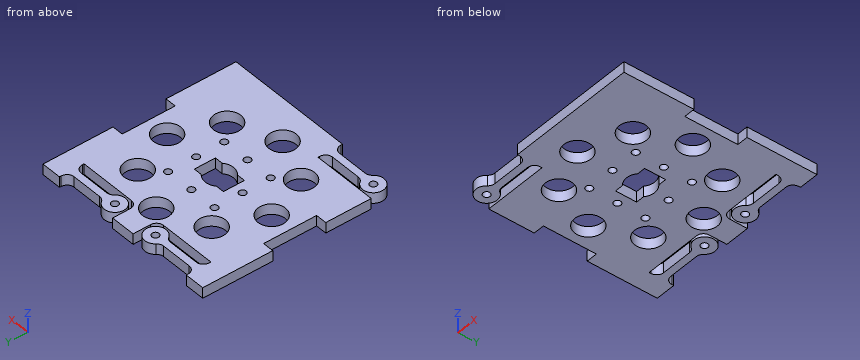
Autodesk Inventor part; units mm, degrees
ref_plane "YZ Plane" through (0, 0, 0) normal (1, 0, 0) x (0, 1, 0)
ref_plane "XZ Plane" through (0, 0, 0) normal (0, 1, 0) x (-1, 0, 0)
ref_plane "XY Plane" through (0, 0, 0) normal (0, 0, 1) x (1, 0, 0)
ref_plane "Work Plane1" through (0, 0, 0) normal (0, 0, 1) x (1, 0, 0)
sketch "Sketch1" plane through (0, 0, 0) normal (0, 0, 1) x (1, 0, 0)
  circle A0 centre (6.5, 20.75) radius 1
  circle A1 centre (6.5, 4.75) radius 1
  circle A2 centre (22.5, 20.75) radius 1
  circle A3 centre (22.5, 4.75) radius 1
  line L0 (-13, -14.75) -> (42, -14.75)
  line L1 (42, -14.75) -> (42, 40.25)
  line L2 (42, 40.25) -> (-13, 40.25)
  line L3 (-13, 40.25) -> (-13, -14.75)
  line L4 (-13, -14.75) -> (42, 40.25) construction
  line L5 (42, -14.75) -> (-13, 40.25) construction
  circle A4 centre (22.5, 12.75) radius 1
  circle A5 centre (14.5, 20.75) radius 1
  circle A6 centre (14.5, 4.75) radius 1
  circle A7 centre (6.5, 12.75) radius 1
  line L6 (19.5, 15.75) -> (19.5, 9.75)
  line L7 (17.1458, 15.75) -> (19.5, 15.75)
  arc A8 (17.1458, 15.75) -> (11.8542, 15.75) centre (14.5, 12.75) ccw
  line L8 (9.5, 15.75) -> (11.8542, 15.75)
  line L9 (9.5, 9.75) -> (9.5, 15.75)
  line L10 (11.8542, 9.75) -> (9.5, 9.75)
  arc A9 (11.8542, 9.75) -> (17.1458, 9.75) centre (14.5, 12.75) ccw
  line L11 (19.5, 9.75) -> (17.1458, 9.75)
  point P0 (0, 0)
  dimension "d0" = 55
  dimension "d1" = 55
  dimension "d95" = 2
  dimension "d96" = 2
  dimension "d97" = 2
  dimension "d98" = 2
extrude "Extrusion3" add sketch "Sketch1" along normal blind 3
sketch "Sketch4" plane through (0, 0, 3) normal (0, 0, 1) x (1, 0, 0)
  line L0 (42, 40.25) -> (-13, 40.25) construction
  line L1 (14.5, 40.25) -> (14.5, 12.75) construction
  line L2 (-13, -14.75) -> (42, -14.75) construction
  line L3 (-13, 40.25) -> (-13, -14.75) construction
  line L4 (-13, 12.75) -> (14.5, 12.75) construction
  circle A0 centre (14.5, 30.75) radius 3.895
  circle A1 centre (1.7721, 25.4779) radius 3.895
  circle A2 centre (-3.5, 12.75) radius 3.895
  circle A3 centre (1.7721, 0.0221) radius 3.895
  circle A4 centre (14.5, -5.25) radius 3.895
  circle A5 centre (27.2279, 0.0221) radius 3.895
  circle A6 centre (32.5, 12.75) radius 3.895
  circle A7 centre (27.2279, 25.4779) radius 3.895
  arc A8 (4.6716, 35.75) -> (4.6716, 37.75) centre (7.5, 36.75) ccw
  line L5 (42, 40.25) -> (-13, 40.25)
  line L6 (7.5, 36.75) -> (-13, 36.75) construction
  line L7 (4.6716, 37.75) -> (-7.3284, 37.75)
  line L8 (4.6716, 35.75) -> (-7.3284, 35.75)
  line L9 (-7.3284, 37.75) -> (-7.3284, 40.25)
  line L10 (10.9716, 40.25) -> (-7.3284, 40.25)
  line L11 (-7.3284, 35.75) -> (-7.3284, 33.25)
  line L12 (-7.3284, 33.25) -> (10.9716, 33.25)
  line L13 (10.9716, 40.25) -> (10.9716, 33.25)
  arc A9 (24.3284, 37.75) -> (24.3284, 35.75) centre (21.5, 36.75) ccw
  line L14 (24.3284, 37.75) -> (36.3284, 37.75)
  line L15 (24.3284, 35.75) -> (36.3284, 35.75)
  line L16 (36.3284, 37.75) -> (36.3284, 40.25)
  line L17 (18.0284, 40.25) -> (36.3284, 40.25)
  line L18 (36.3284, 35.75) -> (36.3284, 33.25)
  line L19 (36.3284, 33.25) -> (18.0284, 33.25)
  line L20 (18.0284, 40.25) -> (18.0284, 33.25)
  arc A10 (-6.6716, -10.25) -> (-6.6716, -12.25) centre (-9.5, -11.25) ccw
  line L21 (-9.5, -11.25) -> (8.4531, -11.25) construction
  line L22 (-6.6716, -10.25) -> (5.3284, -10.25)
  line L23 (-6.6716, -12.25) -> (5.3284, -12.25)
  line L24 (5.3284, -12.25) -> (5.3284, -14.75)
  line L25 (5.3284, -10.25) -> (5.3284, -7.75)
  line L26 (5.3284, -7.75) -> (-13, -7.75)
  line L27 (-13, -14.75) -> (-13, -7.75)
  line L28 (-13, -14.75) -> (5.3284, -14.75)
  point P0 (0, 0)
  dimension "d24" = 7.79
  dimension "d25" = 18
  dimension "d28" = 360
  dimension "d63" = 6
  dimension "d64" = 7
  dimension "d65" = 12
  dimension "d66" = 18.3
  dimension "d67" = 2.5
  dimension "d68" = 3.5
  dimension "d71" = 1
  dimension "d74" = 6
  dimension "d75" = 3.5
  dimension "d76" = 3.5
  dimension "d77" = 12
  dimension "d78" = 1
  dimension "d79" = 2.5
extrude "Extrusion2" cut sketch "Sketch4" against normal through all
hole "Hole4" at (7.5, 36.75, 3) at (21.5, 36.75, 3) at (-9.5, -11.25, 3) direction (0, 0, -1) diameter 2 end through all
fillet "Fillet3" radius 2 14 edges at (-7.3284, 35.75, 1.5) (-7.3284, 37.75, 1.5) (4.6716, 37.75, 1.5) (4.6716, 35.75, 1.5) (10.9716, 33.25, 1.5) (24.3284, 37.75, 1.5) (24.3284, 35.75, 1.5) (36.3284, 37.75, 1.5) (36.3284, 35.75, 1.5) (18.0284, 33.25, 1.5) (5.3284, -10.25, 1.5) (5.3284, -12.25, 1.5) (-6.6716, -10.25, 1.5) (-6.6716, -12.25, 1.5)
sketch "Sketch6" plane through (0, 0, 3) normal (0, 0, 1) x (1, 0, 0)
  line L0 (38.85, 20.3) -> (42, 20.3)
  line L1 (42, 20.3) -> (42, 5.2)
  line L2 (42, 5.2) -> (38.85, 5.2)
  line L3 (38.85, 5.2) -> (38.85, 20.3)
  line L4 (42, -14.75) -> (42, 40.25)
  line L5 (18.0284, 40.25) -> (10.9716, 40.25) construction
  line L6 (14.5, 40.25) -> (14.5, -14.75) construction
  line L7 (5.3284, -14.75) -> (42, -14.75) construction
  line L8 (-9.85, 20.3) -> (-13, 20.3)
  line L9 (-13, 20.3) -> (-13, 5.2)
  line L10 (-13, 5.2) -> (-9.85, 5.2)
  line L11 (-9.85, 5.2) -> (-9.85, 20.3)
  line L12 (-13, -14.75) -> (-13, 40.25)
  point P0 (0, 0)
  point P1 (42, 12.75)
  point P2 (42, 12.75)
  point P3 (-13, 12.75)
  point P4 (-13, 12.75)
  dimension "d91" = 3.15
  dimension "d92" = 15.1
extrude "Extrusion4" cut sketch "Sketch6" against normal through all
equation "\"d38\" = d24"
properties part number "Bottom"
Geometry: final body of the model. Coordinates: model frame, mm. Round coordinates to 2 decimals unless told otherwise and drop trailing zeros. Order: outer loops, then holes, each group sorted by start corner. A loop starts at its lowest first (then second) coordinate and runs counter-clockwise, first axis right, second up. Notation, with made-up numbers: (44, 47.25) -> (50, 47.25) arc R12 cw to (50, 64.25) -> close; hole circle Ø2 at (-35, 55). An arc over 180 degrees is marked (long way). Use CSV: the item, a comma, the result in double quotes. Start each with the question number.
1) Section C-C (x = -3.5). Return the cut outline in (y, z) (3 decimals), and give its area (3 significant figures).
2) Section A-A (y = 30.75). Return the cut outline in (x, z) (3 decimals).
3) Section B-B (x = 14.5). Return the cut outline in (y, z) (3 decimals), and give its area (3 significant figures).
4) Material intervals for line 1 along Y through (x, z) = (5, 2.15); line 2 along Y through (x, z) = (32.5, 1.6) (3 decimals); line 3 along Y through (x, z) = (14.5, 2.2) (3 decimals), sorted ascending. Write a range as from..to.
5) First-contact query: pin 1 Ø12 at (x, y) = (-4, 27) entering from -Z; pin 2 Ø1.5 at (x, z) = (7, 2.5) entering from +Y; pin 3 Ø1.5 at (x, z) = (1, 2) entering from +Y. Flat tips, straight axial feed; report the tip coordinate or a pass-through.
6) Section D-D (y = 36.75). Return the cut outline in (x, z), and give its area (3 significant figures).
Returned:
1,outline,"(-12.25, 0) -> (-10.25, 0) -> (-10.25, 3) -> (-12.25, 3) -> close; (-7.75, 0) -> (8.855, 0) -> (8.855, 3) -> (-7.75, 3) -> close; (16.645, 0) -> (33.25, 0) -> (33.25, 3) -> (16.645, 3) -> close; (35.75, 0) -> (37.75, 0) -> (37.75, 3) -> (35.75, 3) -> close"
1,area,"112 mm²"
2,outline,"(-13, 0) -> (10.605, 0) -> (10.605, 3) -> (-13, 3) -> close; (18.395, 0) -> (42, 0) -> (42, 3) -> (18.395, 3) -> close"
3,outline,"(-14.75, 0) -> (-9.145, 0) -> (-9.145, 3) -> (-14.75, 3) -> close; (-1.355, 0) -> (3.75, 0) -> (3.75, 3) -> (-1.355, 3) -> close; (5.75, 0) -> (8.75, 0) -> (8.75, 3) -> (5.75, 3) -> close; (16.75, 0) -> (19.75, 0) -> (19.75, 3) -> (16.75, 3) -> close; (21.75, 0) -> (26.855, 0) -> (26.855, 3) -> (21.75, 3) -> close; (34.645, 0) -> (40.25, 0) -> (40.25, 3) -> (34.645, 3) -> close"
3,area,"82.3 mm²"
4,line 1,"y = -13.15..-9.35, -7.75..-2.16, 2.2..23.3, 27.66..33.25, 35.07..38.43"
4,line 2,"y = -14.75..8.855, 16.645..33.25, 35.75..37.75"
4,line 3,"y = -14.75..-9.145, -1.355..3.75, 5.75..8.75, 16.75..19.75, 21.75..26.855, 34.645..40.25"
5,pin 1,"stops at z = 0"
5,pin 2,"stops at y = 39.75"
5,pin 3,"stops at y = 37.75"
6,outline,"(-13, 0) -> (6.5, 0) -> (6.5, 3) -> (-13, 3) -> close; (8.5, 0) -> (10.5, 0) -> (10.5, 3) -> (8.5, 3) -> close; (10.97, 0) -> (18.03, 0) -> (18.03, 3) -> (10.97, 3) -> close; (18.5, 0) -> (20.5, 0) -> (20.5, 3) -> (18.5, 3) -> close; (22.5, 0) -> (42, 0) -> (42, 3) -> (22.5, 3) -> close"
6,area,"150 mm²"
